from build123d import *

# Parameters (mm, degrees)
SKETCH1_W            = 95
SKETCH1_H            = 48.2
BOSS_EXTRUDE2_DEPTH  = 1.7
SKETCH3_W            = 92.3
SKETCH3_H            = 45.4
BOSS_EXTRUDE3_DEPTH  = 4.8
SKETCH4_W            = 87.05
SKETCH4_H            = 42.3
CUT_EXTRUDE1_DEPTH   = 7.5
CHAMFER1_SIZE        = 0.96
CHAMFER2_SIZE        = 0.96
CHAMFER3_SIZE        = 0.96
CHAMFER4_SIZE        = 0.96
CHAMFER5_SIZE        = 6.31
CHAMFER5_SIZE2       = 1.51
CHAMFER6_SIZE        = 6.31
CHAMFER6_SIZE2       = 1.51
SKETCH5_W            = 92.3
SKETCH5_H            = 40.2
BOSS_EXTRUDE11_DEPTH = 11.5
SKETCH6_W            = 90.5
SKETCH6_H            = 40.2
CUT_EXTRUDE2_DEPTH   = 11.5
SKETCH7_W            = 92.3
SKETCH7_H            = 40.2
BOSS_EXTRUDE12_DEPTH = 1.2
SKETCH8_W            = 87.3
SKETCH8_H            = 40.2
CUT_EXTRUDE3_DEPTH   = 1.2


with BuildPart() as part:
    # Sketch1 → Boss-Extrude2 (new body)
    with BuildSketch(Plane(origin=(0, 0, 0), x_dir=(1, 0, 0), z_dir=(0, 1, 0))):
        Rectangle(SKETCH1_W, SKETCH1_H)
    extrude(amount=BOSS_EXTRUDE2_DEPTH)

    # Sketch3 → Boss-Extrude3 (add)
    with BuildSketch(Plane(origin=(0, 1.7, 0), x_dir=(1, 0, 0), z_dir=(0, 1, 0))):
        Rectangle(SKETCH3_W, SKETCH3_H)
    extrude(amount=BOSS_EXTRUDE3_DEPTH)

    # Sketch4 → Cut-Extrude1 (cut, through all)
    with BuildSketch(Plane(origin=(0, 6.5, 0), x_dir=(-1, 0, 0), z_dir=(0, 1, 0))):
        Rectangle(SKETCH4_W, SKETCH4_H)
    extrude(amount=-CUT_EXTRUDE1_DEPTH, mode=Mode.SUBTRACT)

    # Chamfer1
    chamfer1_edges = [part.edges().sort_by_distance(p)[0] for p in [
        (47.5, 0, 0),
    ]]
    chamfer(chamfer1_edges, length=CHAMFER1_SIZE)

    # Chamfer2
    chamfer2_edges = [part.edges().sort_by_distance(p)[0] for p in [
        (-0.48, 0, -24.1),
    ]]
    chamfer(chamfer2_edges, length=CHAMFER2_SIZE)

    # Chamfer3
    chamfer3_edges = [part.edges().sort_by_distance(p)[0] for p in [
        (-47.5, 0, 0.48),
    ]]
    chamfer(chamfer3_edges, length=CHAMFER3_SIZE)

    # Chamfer4
    chamfer4_edges = [part.edges().sort_by_distance(p)[0] for p in [
        (0, 0, 24.1),
    ]]
    chamfer(chamfer4_edges, length=CHAMFER4_SIZE)

    # Chamfer5
    chamfer5_edges = [part.edges().sort_by_distance(p)[0] for p in [
        (-43.525, 0, 0),
    ]]
    chamfer5_side = [part.faces().sort_by_distance(p)[0] for p in [
        (-43.525, 3.25, 0),
    ]]
    chamfer(chamfer5_edges, length=CHAMFER5_SIZE, length2=CHAMFER5_SIZE2, reference=chamfer5_side[0])

    # Chamfer6
    chamfer6_edges = [part.edges().sort_by_distance(p)[0] for p in [
        (43.525, 0, 0),
    ]]
    chamfer6_side = [part.faces().sort_by_distance(p)[0] for p in [
        (43.525, 3.25, 0),
    ]]
    chamfer(chamfer6_edges, length=CHAMFER6_SIZE, length2=CHAMFER6_SIZE2, reference=chamfer6_side[0])

    # Sketch5 → Boss-Extrude11 (add)
    with BuildSketch(Plane(origin=(0, 6.5, 0), x_dir=(1, 0, 0), z_dir=(0, 1, 0))):
        Rectangle(SKETCH5_W, SKETCH5_H)
    extrude(amount=BOSS_EXTRUDE11_DEPTH)

    # Sketch6 → Cut-Extrude2 (cut)
    with BuildSketch(Plane(origin=(0, 18, 0), x_dir=(1, 0, 0), z_dir=(0, 1, 0))):
        Rectangle(SKETCH6_W, SKETCH6_H)
    extrude(amount=-CUT_EXTRUDE2_DEPTH, mode=Mode.SUBTRACT)

    # Sketch7 → Boss-Extrude12 (add)
    with BuildSketch(Plane(origin=(0, 18, 0), x_dir=(-1, 0, 0), z_dir=(0, 1, 0))):
        Rectangle(SKETCH7_W, SKETCH7_H)
    extrude(amount=BOSS_EXTRUDE12_DEPTH)

    # Sketch8 → Cut-Extrude3 (cut)
    with BuildSketch(Plane(origin=(0, 19.2, 0), x_dir=(1, 0, 0), z_dir=(0, 1, 0))):
        Rectangle(SKETCH8_W, SKETCH8_H)
    extrude(amount=-CUT_EXTRUDE3_DEPTH, mode=Mode.SUBTRACT)


solid = part.part
Geometry: final body of the model. Coordinates: model frame, mm. A direction names the side the tool comes from. Coordinates: 2 decimals unless noted, no trailing zeros. Loops run counter-clockwise (first coordinate to the right, second up) from the corner with the lowest first, then second, coordinate; pieces in that order, holes last. Notation, with made-up numbers: (-9.5, 15) - (32.5, 15) arc R8 ccw to (32.5, 22) - close; hole circle Ø7 at (72, 53). An arc over 180 degrees is marked (long way). Put each result on its own line as item: value. Start each with the question number.
Q1. Pin query (flat end, axial travel): pin 1 Ø2.5 at (x, y) = (17, 4) entering from +Z; pin 2 Ø1.2 at (x, y) = (45, 11.5) entering from +Z; pin 3 Ø5 at (y, z) = (9.5, -2) entering from +X. Return the tip coordinate at first contact, or that it passes through.
Q2. Cut plane B-B, the plane z = 4. Return loops of the section in (x, y) (3 decimals), and give its area (3 significant figures).
Q3. Cut plane A-A, the plane x = 5. Return loops of the section in (y, z).
Q4. Cut plane D-D, the plane y = 3. Return loops of the section in (x, z), and give its area (3 significant figures).
Q5. Line query: line 1 (X direction, y = 6.75, z = 9); line 2 (Z direction, x = -2, y = 2); line 3 (X direction, y = 18.5, z = -5). Output: solid intervals per line, ascending.
Q6. Pull-direction query (Y, two-part tool) for faces 1 (the flat face through (-4, 6.5, 22)), 2 (the flat face through (45.25, 12, 0)), 3 (the flat face through (0, 0, -22)), 4 (the flat face through (46.15, 10, 0)); classes: released by +Y, released by -Y, zero draft, split by the parting line, or undercut.
Q7. Set-up query: faces 5 (the flat face through (44.29, 3.11, -0.3)), 6 (the flat face through (-45.44, 14.17, -20.1)), 7 (the flat face through (-45.25, 12, 0)), 8 (the flat face through (-45.44, 14.17, 20.1)), 9 (the flat face through (-46.15, 10, 0)). Return all of +Z, -Z, +X, -X, +Y, -Y with unobstructed straight access to the full face (end or side cutting, diameter ignored); none if empty.
Q8. Cut plane C-C, the plane y = 14.25. Return loops of the section in (x, z), and give its area (3 significant figures).
Filled sheet:
1. pin 1: z = 22.7
1. pin 2: z = 20.1
1. pin 3: x = 46.15
2. outline: (-47.5, 0.96) - (-46.54, 0) - (-45.035, 0) - (-43.525, 6.31) - (-43.525, 6.5) - (-45.25, 6.5) - (-45.25, 18) - (-43.65, 18) - (-43.65, 19.2) - (-46.15, 19.2) - (-46.15, 1.7) - (-47.5, 1.7) - close; (43.525, 6.31) - (45.035, 0) - (46.54, 0) - (47.5, 0.96) - (47.5, 1.7) - (46.15, 1.7) - (46.15, 19.2) - (43.65, 19.2) - (43.65, 18) - (45.25, 18) - (45.25, 6.5) - (43.525, 6.5) - close
2. area: 55.0 mm²
3. outline: (0, -23.14) - (0.96, -24.1) - (1.7, -24.1) - (1.7, -22.7) - (6.5, -22.7) - (6.5, -21.15) - (0, -21.15) - close; (0, 21.15) - (6.5, 21.15) - (6.5, 22.7) - (1.7, 22.7) - (1.7, 24.1) - (0.96, 24.1) - (0, 23.14) - close
4. outline: (-46.15, -22.7) - (46.15, -22.7) - (46.15, 22.7) - (-46.15, 22.7) - close; hole (-44.32, -21.15) - (44.32, -21.15) - (44.32, 21.15) - (-44.32, 21.15) - close
4. area: 441 mm²
5. line 1: -46.15 to -45.25, 45.25 to 46.15
5. line 2: -22.7 to -21.15, 21.15 to 22.7
5. line 3: -46.15 to -43.65, 43.65 to 46.15
6. face 1: undercut
6. face 2: undercut
6. face 3: released by -Y
6. face 4: zero draft
7. face 5: -Y
7. face 6: -Z, +X, -X, +Y
7. face 7: +Z, -Z
7. face 8: +Z, +X, -X, +Y
7. face 9: +Z, -Z, -X, +Y
8. outline: (-46.15, -20.1) - (-45.25, -20.1) - (-45.25, 20.1) - (-46.15, 20.1) - close; (45.25, -20.1) - (46.15, -20.1) - (46.15, 20.1) - (45.25, 20.1) - close
8. area: 72.4 mm²
